Autodesk Inventor part; units mm, degrees
ref_plane "YZ Plane" through (0, 0, 0) normal (1, 0, 0) x (0, 1, 0)
ref_plane "XZ Plane" through (0, 0, 0) normal (0, 1, 0) x (-1, 0, 0)
ref_plane "XY Plane" through (0, 0, 0) normal (0, 0, 1) x (1, 0, 0)
sketch "Sketch1" plane through (0, 0, 0) normal (0, 0, 1) x (1, 0, 0)
  line L0 (-7, -3) -> (7, -3)
  line L1 (7, -3) -> (7, 3)
  line L2 (7, 3) -> (-7, 3)
  line L3 (-7, 3) -> (-7, -3)
  line L4 (-7, -3) -> (7, 3) construction
  line L5 (7, -3) -> (-7, 3) construction
  point P0 (0, 0)
  dimension "d0" = 14
  dimension "d1" = 6
extrude "Extrusion1" add sketch "Sketch1" along normal blind 10
sketch "Sketch2" plane through (0, 0, 10) normal (0, 0, 1) x (1, 0, 0)
  line L0 (-2.5, 0) -> (-2.5, 3)
  line L1 (7, 3) -> (-7, 3)
  line L2 (-2.5, 0) -> (-2.5, -3)
  line L3 (-7, -3) -> (7, -3)
  line L4 (2.5, 0) -> (2.5, 3)
  line L5 (2.5, 0) -> (2.5, -3)
  point P0 (0, 0)
extrude "Extrusion2" cut sketch "Sketch2" against normal blind 7.5
properties part number "opto"
Here's how the part is built. I have some questions about the finished solid (model axes, mm). A direction names the side the tool comes from. Give positions to 0.01 mm unless a question says otherwise; leave off trailing zeros. Order: outer loops, then holes, each group sorted by start corner. A loop starts at its lowest first (then second) coordinate and runs counter-clockwise, first axis right, second up. Notation, with made-up numbers: (70.25, 88) -> (105.25, 88) arc R28 ccw to (105.25, 112) -> close; hole circle Ø1 at (-30, 87). An arc over 180 degrees is marked (long way). Use CSV: the item, a comma, the result in double quotes. Start each with the question number.
Item 1: If I drill on probe 1 along X at (y, z) = (-2.2, 6.5); probe 2 along Z at (x, y) = (1, -0.75), over which ranges is the centre line in solid material (lowest first)? Write a range as [from, to].
Item 2: Thinking about a two-plate mould opening in X: for faces 3 (the flat face through (-2.5, 0, 6)), 4 (the flat face through (-7, 0, 5)), 5 (the flat face through (0, 0, 0)), which applies, pulls with the +X half, pulls with the -X half, needs draft (parallel to the pull), parting line crosses it, or undercut?
Item 3: Suppose I cut it at B-B (y = 0.8). List the corners of the cut face in (x, z) for me.
Item 4: On a 3-axis mill with a long thin cutter (end or side, diameter ignored), from which of +Z, -Z, +X, -X, +Y, -Y can I reach the whole of each face in a straight line? I mean faces 1 (the flat face through (2.5, 0, 6)), 2 (the flat face through (-5, 0, 10)). Say none if no direction works.
Item 5: I'm going to push a flat-ended pin straight in: P1, Ø1.5, axis at x = 1, y = 1.5, coming from the +Z side. Where does the tip first touch, or does it pass through?
Item 6: Suppose I cut it at C-C (x = 1.75). List the corners of the cut face in (y, z) for me.
Item 7: Suppose I cut it at A-A (z = 4). List the corners of the cut face in (x, y) for me, and give its area (3 significant figures).
Answer block:
1,probe 1,"x = [-7, -2.5], [2.5, 7]"
1,probe 2,"z = [0, 2.5]"
2,face 3,"undercut"
2,face 4,"pulls with the -X half"
2,face 5,"needs draft"
3,outline,"(-7, 0) -> (7, 0) -> (7, 10) -> (2.5, 10) -> (2.5, 2.5) -> (-2.5, 2.5) -> (-2.5, 10) -> (-7, 10) -> close"
4,face 1,"+Z, +Y, -Y"
4,face 2,"+Z, +X, -X, +Y, -Y"
5,P1,"stops at z = 2.5"
6,outline,"(-3, 0) -> (3, 0) -> (3, 2.5) -> (-3, 2.5) -> close"
7,outline,"(-7, -3) -> (-2.5, -3) -> (-2.5, 3) -> (-7, 3) -> close; (2.5, -3) -> (7, -3) -> (7, 3) -> (2.5, 3) -> close"
7,area,"54.0 mm^2"
